Design review of the part built by this model. Coordinates are the model's own, in mm. Face numbers are marked on the shaded views. A direction names the side the tool comes from. Give positions to 0.01 mm unless a question says otherwise; leave off trailing zeros. Use a Markdown table: item, result. Add a question column.
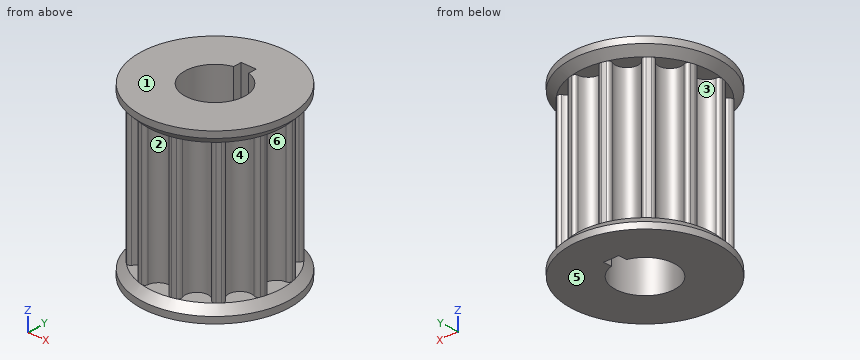
```python
from build123d import *

# Parameters (mm, degrees)
SALIENTE_EXTRUIR1_DEPTH   = 9.25
CROQUIS5_R                = 8.98
SALIENTE_EXTRUIR2_DEPTH   = 1
SALIENTE_EXTRUIR2_DRAFT   = -45
CROQUIS8_R                = 9.98
SALIENTE_EXTRUIR3_DEPTH   = 0.86250003
SIMETR_A1_COPY_1_SKETCH_R = 8.98
SIMETR_A1_COPY_1_DEPTH    = 1
SIMETR_A1_COPY_1_DRAFT    = -45
CORTAR_EXTRUIR1_DEPTH     = 27.327769136


with BuildPart() as part:
    # Croquis3 → Saliente-Extruir1 (new, symmetric)
    with BuildSketch(Plane.XY):
        with BuildLine():
            ThreePointArc((0, 6.92), (1.044537818, 7.333889859), (1.522093853, 8.350897382))
            ThreePointArc((1.522093853, 8.350897382), (1.69468698, 8.669418435), (2.049408684, 8.74301573))
            ThreePointArc((2.049408684, 8.74301573), (2.324195025, 8.67401392), (2.596667882, 8.596378069))
            ThreePointArc((2.596667882, 8.596378069), (2.867067241, 8.355280091), (2.857276747, 7.993136203))
            ThreePointArc((2.857276747, 7.993136203), (2.762348644, 6.873603835), (3.46, 5.992895794))
            ThreePointArc((3.46, 5.992895794), (4.571541215, 5.829066017), (5.493620634, 6.47104235))
            ThreePointArc((5.493620634, 6.47104235), (5.802351194, 6.660593111), (6.146347848, 6.546969386))
            ThreePointArc((6.146347848, 6.546969386), (6.349818895, 6.349818895), (6.546969386, 6.146347848))
            ThreePointArc((6.546969386, 6.146347848), (6.660593111, 5.802351194), (6.47104235, 5.493620634))
            ThreePointArc((6.47104235, 5.493620634), (5.829066017, 4.571541215), (5.992895794, 3.46))
            ThreePointArc((5.992895794, 3.46), (6.873603835, 2.762348644), (7.993136203, 2.857276747))
            ThreePointArc((7.993136203, 2.857276747), (8.355280091, 2.867067241), (8.596378069, 2.596667882))
            ThreePointArc((8.596378069, 2.596667882), (8.67401392, 2.324195025), (8.74301573, 2.049408684))
            ThreePointArc((8.74301573, 2.049408684), (8.669418435, 1.69468698), (8.350897382, 1.522093853))
            ThreePointArc((8.350897382, 1.522093853), (7.333889859, 1.044537818), (6.92, 0))
            ThreePointArc((6.92, 0), (7.333889859, -1.044537818), (8.350897382, -1.522093853))
            ThreePointArc((8.350897382, -1.522093853), (8.669418435, -1.69468698), (8.74301573, -2.049408684))
            ThreePointArc((8.74301573, -2.049408684), (8.67401392, -2.324195025), (8.596378069, -2.596667882))
            ThreePointArc((8.596378069, -2.596667882), (8.355280091, -2.867067241), (7.993136203, -2.857276747))
            ThreePointArc((7.993136203, -2.857276747), (6.873603835, -2.762348644), (5.992895794, -3.46))
            ThreePointArc((5.992895794, -3.46), (5.829066017, -4.571541215), (6.47104235, -5.493620634))
            ThreePointArc((6.47104235, -5.493620634), (6.660593111, -5.802351194), (6.546969386, -6.146347848))
            ThreePointArc((6.546969386, -6.146347848), (6.349818895, -6.349818895), (6.146347848, -6.546969386))
            ThreePointArc((6.146347848, -6.546969386), (5.802351194, -6.660593111), (5.493620634, -6.47104235))
            ThreePointArc((5.493620634, -6.47104235), (4.571541215, -5.829066017), (3.46, -5.992895794))
            ThreePointArc((3.46, -5.992895794), (2.762348644, -6.873603835), (2.857276747, -7.993136203))
            ThreePointArc((2.857276747, -7.993136203), (2.867067241, -8.355280091), (2.596667882, -8.596378069))
            ThreePointArc((2.596667882, -8.596378069), (2.324195025, -8.67401392), (2.049408684, -8.74301573))
            ThreePointArc((2.049408684, -8.74301573), (1.69468698, -8.669418435), (1.522093853, -8.350897382))
            ThreePointArc((1.522093853, -8.350897382), (1.044537818, -7.333889859), (0, -6.92))
            ThreePointArc((0, -6.92), (-1.044537818, -7.333889859), (-1.522093853, -8.350897382))
            ThreePointArc((-1.522093853, -8.350897382), (-1.69468698, -8.669418435), (-2.049408684, -8.74301573))
            ThreePointArc((-2.049408684, -8.74301573), (-2.324195025, -8.67401392), (-2.596667882, -8.596378069))
            ThreePointArc((-2.596667882, -8.596378069), (-2.867067241, -8.355280091), (-2.857276747, -7.993136203))
            ThreePointArc((-2.857276747, -7.993136203), (-2.762348644, -6.873603835), (-3.46, -5.992895794))
            ThreePointArc((-3.46, -5.992895794), (-4.571541215, -5.829066017), (-5.493620634, -6.47104235))
            ThreePointArc((-5.493620634, -6.47104235), (-5.802351194, -6.660593111), (-6.146347848, -6.546969386))
            ThreePointArc((-6.146347848, -6.546969386), (-6.349818895, -6.349818895), (-6.546969386, -6.146347848))
            ThreePointArc((-6.546969386, -6.146347848), (-6.660593111, -5.802351194), (-6.47104235, -5.493620634))
            ThreePointArc((-6.47104235, -5.493620634), (-5.829066017, -4.571541215), (-5.992895794, -3.46))
            ThreePointArc((-5.992895794, -3.46), (-6.873603835, -2.762348644), (-7.993136203, -2.857276747))
            ThreePointArc((-7.993136203, -2.857276747), (-8.355280091, -2.867067241), (-8.596378069, -2.596667882))
            ThreePointArc((-8.596378069, -2.596667882), (-8.67401392, -2.324195025), (-8.74301573, -2.049408684))
            ThreePointArc((-8.74301573, -2.049408684), (-8.669418435, -1.69468698), (-8.350897382, -1.522093853))
            ThreePointArc((-8.350897382, -1.522093853), (-7.333889859, -1.044537818), (-6.92, 0))
            ThreePointArc((-6.92, 0), (-7.333889859, 1.044537818), (-8.350897382, 1.522093853))
            ThreePointArc((-8.350897382, 1.522093853), (-8.669418435, 1.69468698), (-8.74301573, 2.049408684))
            ThreePointArc((-8.74301573, 2.049408684), (-8.67401392, 2.324195025), (-8.596378069, 2.596667882))
            ThreePointArc((-8.596378069, 2.596667882), (-8.355280091, 2.867067241), (-7.993136203, 2.857276747))
            ThreePointArc((-7.993136203, 2.857276747), (-6.873603835, 2.762348644), (-5.992895794, 3.46))
            ThreePointArc((-5.992895794, 3.46), (-5.829066017, 4.571541215), (-6.47104235, 5.493620634))
            ThreePointArc((-6.47104235, 5.493620634), (-6.660593111, 5.802351194), (-6.546969386, 6.146347848))
            ThreePointArc((-6.546969386, 6.146347848), (-6.349818895, 6.349818895), (-6.146347848, 6.546969386))
            ThreePointArc((-6.146347848, 6.546969386), (-5.802351194, 6.660593111), (-5.493620634, 6.47104235))
            ThreePointArc((-5.493620634, 6.47104235), (-4.571541215, 5.829066017), (-3.46, 5.992895794))
            ThreePointArc((-3.46, 5.992895794), (-2.762348644, 6.873603835), (-2.857276747, 7.993136203))
            ThreePointArc((-2.857276747, 7.993136203), (-2.867067241, 8.355280091), (-2.596667882, 8.596378069))
            ThreePointArc((-2.596667882, 8.596378069), (-2.324195025, 8.67401392), (-2.049408684, 8.74301573))
            ThreePointArc((-2.049408684, 8.74301573), (-1.69468698, 8.669418435), (-1.522093853, 8.350897382))
            ThreePointArc((-1.522093853, 8.350897382), (-1.044537818, 7.333889859), (0, 6.92))
        make_face()
    extrude(amount=SALIENTE_EXTRUIR1_DEPTH, both=True)


with BuildPart() as saliente_extruir2_tool:
    # Croquis5 → Saliente-Extruir2 (with draft: the straight prism first)
    with BuildSketch(Plane.XY.offset(9.25)):
        Circle(CROQUIS5_R)
    extrude(amount=SALIENTE_EXTRUIR2_DEPTH)
    # Saliente-Extruir2: the draft: its side faces are tilted about the plane it starts from
    saliente_extruir2_sides = [saliente_extruir2_tool.faces().sort_by_distance(p)[0] for p in [
        (-8.98, 0, 9.75),
    ]]
    draft(saliente_extruir2_sides, Plane.XY.offset(9.25), SALIENTE_EXTRUIR2_DRAFT)


with BuildPart() as part_1:
    add(part.part)

    # Saliente-Extruir2: add saliente_extruir2_tool
    add(saliente_extruir2_tool.part)

    # Croquis8 → Saliente-Extruir3 (add)
    with BuildSketch(Plane.XY.offset(10.25)):
        Circle(CROQUIS8_R)
    saliente_extruir3 = extrude(amount=SALIENTE_EXTRUIR3_DEPTH)


with BuildPart() as simetr_a1_1:
    # Simetr_a1: Saliente-Extruir3 across plane
    add(saliente_extruir3.mirror(Plane.XY))


with BuildPart() as simetr_a1_copy_1_tool:
    # Simetr_a1 copy 1 sketch → Simetr_a1 copy 1 (with draft: the straight prism first)
    with BuildSketch(Plane(origin=(0, 0, -9.25), x_dir=(1, 0, 0), z_dir=(0, 0, -1))):
        Circle(SIMETR_A1_COPY_1_SKETCH_R)
    extrude(amount=SIMETR_A1_COPY_1_DEPTH)
    # Simetr_a1 copy 1: the draft: its side faces are tilted about the plane it starts from
    simetr_a1_copy_1_sides = [simetr_a1_copy_1_tool.faces().sort_by_distance(p)[0] for p in [
        (-8.98, 0, -9.75),
    ]]
    draft(simetr_a1_copy_1_sides, Plane(origin=(0, 0, -9.25), x_dir=(1, 0, 0), z_dir=(0, 0, -1)), SIMETR_A1_COPY_1_DRAFT)


with BuildPart() as part_2:
    add(part_1.part)

    # Simetr_a1 copy 1: add simetr_a1_copy_1_tool
    add(simetr_a1_copy_1_tool.part)

    add(simetr_a1_1.part)  # Simetr_a1 copy 1 merges Simetr_a1_1

    # Croquis6 → Cortar-Extruir1 (cut, through all)
    with BuildSketch(Plane.XY.offset(11.11250003)):
        with BuildLine():
            Line((-1.035, 3.889652941), (-1.035, 5.04))
            Line((-1.035, 5.04), (1.035, 5.04))
            Line((1.035, 5.04), (1.035, 3.889652941))
            ThreePointArc((1.035, 3.889652941), (0, -4.025), (-1.035, 3.889652941))
        make_face()
    extrude(amount=-CORTAR_EXTRUIR1_DEPTH, mode=Mode.SUBTRACT)


solid = part_2.part
```
(1) Tool access review of the marked faces 4, 5 and 6: name each direction out of +Z, -Z, +X, -X, +Y, -Y from which nothing blocks a thin tool from reaching the whole face with its end or side.
(2) Mouldability with a two-part tool opening along Y and no side actions: class the marked faces 1, 2 and 3 as +Y half, -Y half, draft (parallel to the pull), parting line (faces both ways), or undercut.
(3) Insertion check: pin 1 (5 mm diameter, centred on y = -4, z = -1.5, fed in from -X); pin 2 (0.6 mm diameter, centred on x = -0.5, z = 2, fed in from -Y); pin 3 (2 mm diameter, centred on x = -3, z = -6, fed in from -Y). Each pin has a flat end and moves straight along its axis. Give the tip position at first contact, or say it passes through.
(4) For line 1 along Y through (x, z) = (0, -3.5) (3 decimals); line 2 along X through (y, z) = (-6, -1.75); line 3 along Z through (x, y) = (7, 4.5), list the stretches that pass through material, from the lowest coordinate up.
Answers follow:
| question | item | result |
|---|---|---|
| 1 | face 4 | none |
| 1 | face 5 | -Z, +X, -X, +Y, -Y |
| 1 | face 6 | +X |
| 2 | face 1 | draft |
| 2 | face 2 | -Y half |
| 2 | face 3 | undercut |
| 3 | pin 1 | x = -8.75 |
| 3 | pin 2 | y = -7.15 |
| 3 | pin 3 | y = -8.75 |
| 4 | line 1 | -6.92 to -4.025, 5.04 to 6.92 |
| 4 | line 2 | -6.64 to -5, -3.45 to 3.45, 5 to 6.64 |
| 4 | line 3 | -11.11 to -9.25, 9.25 to 11.11 |
